Could you check a few things on this model? Use its own coordinates, in mm. Face numbers are marked on the shaded views. A direction names the side the tool comes from. Give positions to 0.01 mm unless a question says otherwise; leave off trailing zeros. Loops run counter-clockwise (first coordinate to the right, second up) from the corner with the lowest first, then second, coordinate; pieces in that order, holes last. Notation, with made-up numbers: (30.5, 52.25) - (56.5, 52.25) arc R24 ccw to (56.5, 68.25) - close; hole circle Ø10 at (87.25, -14.5). An arc over 180 degrees is marked (long way). Write each question's results on one line, items separated by ' | '. Start each with the question number.
1) I want a section at B-B, the plane y = 0. Write out the boundary of the cut face in (x, z).
2) I want a section at D-D, the plane x = -6. Write out the boundary of the cut face in (y, z) (3 decimals).
3) I'm going to push flat-ended pins straight in: pin 1 (8 mm diameter, centred on x = 10, y = -57.5, fed in from -Z); pin 2 (8 mm diameter, centred on y = -71, z = -6, fed in from +X); pin 3 (4 mm diameter, centred on y = -100, z = -7.5, fed in from -X); pin 4 (1.5 mm diameter, centred on y = -40.5, z = -19, fed in from -X). Where does each tip first touch, or does it pass through?
4) I want a section at C-C, the plane z = 4.5. Write out the boundary of the cut face in (x, y).
5) On a 3-axis mill with a long thin cutter (end or side, diameter ignored), from which of +Z, -Z, +X, -X, +Y, -Y can I reach the whole of each face in a straight line? I mean the marked faces 1 and 2. Say none if no direction works.
6) If I drill on probe 1 along Z at (x, y) = (7.5, 10); probe 2 along X at (y, z) = (-105, -11); probe 3 along X at (y, z) = (-73, -6.5), over which ranges is the centre line in solid material (lowest first)? Write a range as [from, to].
7) I want a section at A-A, the plane x = 9. Write out the boundary of the cut face in (y, z) (3 decimals).
from build123d import *

# Parameters (mm, degrees)
SKETCH1_R           = 19.05
BOSS_EXTRUDE1_DEPTH = 12.7
BOSS_EXTRUDE2_START = -12.7
BOSS_EXTRUDE2_DEPTH = 12.7
BOSS_EXTRUDE3_DEPTH = 26.035


with BuildPart() as part:
    # Sketch1 → Boss-Extrude1 (new body)
    with BuildSketch(Plane.XY):
        Circle(SKETCH1_R)
    extrude(amount=BOSS_EXTRUDE1_DEPTH)

    # Sketch2 → Boss-Extrude2 (add)
    with BuildSketch(Plane.XY.offset(12.7).offset(BOSS_EXTRUDE2_START)):
        with BuildLine():
            Line((-18.887735318, -2.481119615), (-3.587497693, -118.955487411))
            Line((-3.587497693, -118.955487411), (12.152281739, -116.887887732))
            Line((12.152281739, -116.887887732), (-0.701538954, -19.037078113))
            ThreePointArc((-0.701538954, -19.037078113), (-12.824190309, -14.08696713), (-18.887735318, -2.481119615))
        make_face()
    extrude(amount=BOSS_EXTRUDE2_DEPTH)

    # Sketch3 → Boss-Extrude3 (add)
    with BuildSketch(Plane(origin=(0, 0, 0), x_dir=(-1, 0, 0), z_dir=(0, 0, -1))):
        Polygon((3.587497693, -118.955487411), (-12.152281739, -116.887887732), (-0.573723536, -28.745122913), (15.166055896, -30.812722592), align=None)
    extrude(amount=BOSS_EXTRUDE3_DEPTH)


solid = part.part
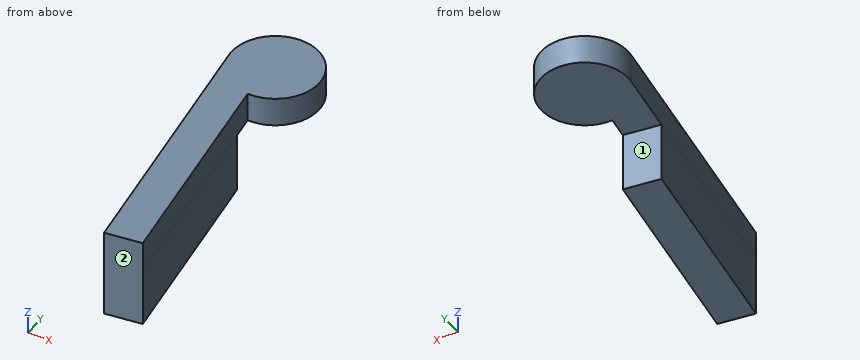
Answers:
1) outline: (-19.05, 0) - (19.05, 0) - (19.05, 12.7) - (-19.05, 12.7) - close
2) outline: (-100.59, -26.035) - (-29.609, -26.035) - (-29.609, 0) - (18.08, 0) - (18.08, 12.7) - (-100.59, 12.7) - close
3) pin 1: passes through | pin 2: stops at x = 6.65 | pin 3: stops at x = -6.34 | pin 4: stops at x = -13.99
4) outline: (-18.89, -2.48) - (-3.59, -118.96) - (12.15, -116.89) - (-0.7, -19.04) arc R19.05 ccw (long way) to start
5) face 1: -Z, -X, +Y | face 2: +Z, -Z, +X, -Y
6) probe 1: z = [0, 12.7] | probe 2: x = [-5.42, 10.59] | probe 3: x = [-9.62, 6.39]
7) outline: (-117.302, -26.035) - (-92.891, -26.035) - (-92.891, 12.7) - (-117.302, 12.7) - close; (-16.79, 0) - (16.79, 0) - (16.79, 12.7) - (-16.79, 12.7) - close
